from build123d import *

# Parameters (mm, degrees)
SKETCH1_W           = 101.6
SKETCH1_H           = 77.47
BOSS_EXTRUDE1_DEPTH = 1.5875
SKETCH2_R           = 1.6002
CUT_EXTRUDE1_DEPTH  = 2.54
SKETCH3_W           = 12.769362992
SKETCH3_H           = 5.005824016
BOSS_EXTRUDE2_DEPTH = 33.274
SKETCH4_W           = 33.664684251
SKETCH4_H           = 48.368799212
BOSS_EXTRUDE3_DEPTH = 10.16
SKETCH5_W           = 15.332321875
SKETCH5_H           = 46.138952111
BOSS_EXTRUDE4_DEPTH = 15.24


with BuildPart() as part:
    # Sketch1 → Boss-Extrude1 (new body)
    with BuildSketch(Plane(origin=(0, 0, 0), x_dir=(1, 0, 0), z_dir=(0, 1, 0))):
        with Locations((-46.570976536, 16.383405637)):
            Rectangle(SKETCH1_W, SKETCH1_H)
    extrude(amount=BOSS_EXTRUDE1_DEPTH)

    # Sketch2 → Cut-Extrude1 (cut)
    with BuildSketch(Plane(origin=(0, 1.5875, 0), x_dir=(1, 0, 0), z_dir=(0, 1, 0))):
        with Locations((-93.560976536, -18.541594363)):
            Circle(SKETCH2_R)
        with Locations((-93.560976536, 51.308405637)):
            Circle(SKETCH2_R)
        with Locations((0.419023464, 51.308405637)):
            Circle(SKETCH2_R)
        with Locations((0.419023464, -18.541594363)):
            Circle(SKETCH2_R)
    extrude(amount=-CUT_EXTRUDE1_DEPTH, mode=Mode.SUBTRACT)

    # Sketch3 → Boss-Extrude2 (add)
    with BuildSketch(Plane(origin=(0, 0, 0), x_dir=(1, 0, 0), z_dir=(0, 1, 0))):
        with Locations((-48.957170631, -19.848682355)):
            Rectangle(SKETCH3_W, SKETCH3_H)
    extrude(amount=BOSS_EXTRUDE2_DEPTH)

    # Sketch4 → Boss-Extrude3 (add)
    with BuildSketch(Plane(origin=(0, 0, 0), x_dir=(1, 0, 0), z_dir=(0, 1, 0))):
        with Locations((-23.385471389, 12.894993304)):
            Rectangle(SKETCH4_W, SKETCH4_H)
    extrude(amount=BOSS_EXTRUDE3_DEPTH)

    # Sketch5 → Boss-Extrude4 (add)
    with BuildSketch(Plane(origin=(0, 0, 0), x_dir=(1, 0, 0), z_dir=(0, 1, 0))):
        with Locations((-66.619550072, 12.54421879)):
            Rectangle(SKETCH5_W, SKETCH5_H)
    extrude(amount=BOSS_EXTRUDE4_DEPTH)


solid = part.part
Geometry: final body of the model. Coordinates: model frame, mm. A direction names the side the tool comes from. Round coordinates to 2 decimals unless told otherwise and drop trailing zeros. Loops run counter-clockwise (first coordinate to the right, second up) from the corner with the lowest first, then second, coordinate; pieces in that order, holes last. Notation, with made-up numbers: M 79,-28 L 96,-28 A11 cw 96,-24 Z; hole C 60,88.5 d2. An arc over 180 degrees is marked long. Put each result on its own line as item: value. Start each with the question number.
(1) Draft query along X for faces 1 (the face through (-95.16, 0.8, -51.38)), 2 (the face through (-55.342, 17, 20)), 3 (the face through (-24, 10.16, -13)). Return one class per face: +X half, -X half, draft (parallel to the pull), parting line (faces both ways), or undercut.
(2) Section query D-D (z = -17.5). Return loops of the section in (x, y).
(3) Section query C-C (x = -72). Return loops of the section in (y, z).
(4) Section query B-B (y = 13.5). Return loops of the section in (x, z), then the cut area to 3 significant figures.
(5) Contact query for flat-ended pins moving along their axis: pin 1 Ø11 at (y, z) = (8.5, -24) entering from -X; pin 2 Ø11 at (y, z) = (10, -22) entering from +X; pin 3 Ø10 at (x, z) = (-73.5, 5) entering from -Y; pin 4 Ø4.5 at (x, y) = (-26.5, 6.5) entering from +Z. Output: stop coordinate, or through.
(6) Section query A-A (y = 5.5). Return loops of the section in (x, z), then the cut area to 3 significant figures.
(7) Set-up query: faces 4 (the face through (-58.953, 8, -12)), 5 (the face through (-67, 8, -35.614)), 6 (the face through (-24, 6, 11.289)). Return all of +Z, -Z, +X, -X, +Y, -Y with unobstructed straight access to the full face (end or side cutting, diameter ignored); none if empty.
(8) Material intervals for line 1 along X through (y, z) = (6, -10); line 2 along Y through (x, z) = (-48.5, -19); line 3 along Z through (x, y) = (-50, 28.5), sorted ascending. Write a range as [from, to].
Findings below:
1. face 1: undercut
1. face 2: -X half
1. face 3: draft
2. outline: M -97.37,0 L 4.23,0 L 4.23,1.59 L -6.55,1.59 L -6.55,10.16 L -40.22,10.16 L -40.22,1.59 L -58.95,1.59 L -58.95,15.24 L -74.29,15.24 L -74.29,1.59 L -97.37,1.59 Z
3. outline: M 0,-55.12 L 1.59,-55.12 L 1.59,-35.61 L 15.24,-35.61 L 15.24,10.53 L 1.59,10.53 L 1.59,22.35 L 0,22.35 Z
4. outline: M -74.29,-35.61 L -58.95,-35.61 L -58.95,10.53 L -74.29,10.53 Z; M -55.34,17.35 L -42.57,17.35 L -42.57,22.35 L -55.34,22.35 Z
4. area: 771 mm2
5. pin 1: stops at x = -74.29
5. pin 2: stops at x = -6.55
5. pin 3: stops at y = 0
5. pin 4: stops at z = 11.29
6. outline: M -74.29,-35.61 L -58.95,-35.61 L -58.95,10.53 L -74.29,10.53 Z; M -55.34,17.35 L -42.57,17.35 L -42.57,22.35 L -55.34,22.35 Z; M -40.22,-37.08 L -6.55,-37.08 L -6.55,11.29 L -40.22,11.29 Z
6. area: 2,400 mm2
7. face 4: +Z, -Z, +Y
7. face 5: -Z, -X, +Y
7. face 6: +Z, +X, -X, +Y
8. line 1: x = [-74.29, -58.95], [-40.22, -6.55]
8. line 2: y = [0, 1.59]
8. line 3: z = [17.35, 22.35]
